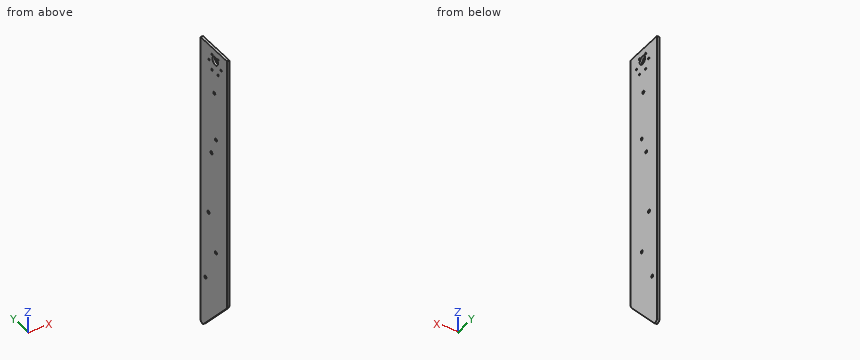
from build123d import *

# Parameters (mm, degrees)
SKETCH_1_R      = 2.5
SKETCH_1_R_2    = 7
SKETCH_1_R_3    = 1.6
EXTRUDE_1_DEPTH = 4


with BuildPart() as part:
    # 草图1 → 凸台-拉伸1 (new body)
    with BuildSketch(Plane.ZY):
        with BuildLine():
            Line((-207.252247772, -7.404631077), (226.406668198, -7.404631077))
            Line((226.406668198, -7.404631077), (226.406668198, 59.595368923))
            Line((226.406668198, 59.595368923), (-273.593331802, 59.595368923))
            ThreePointArc((-273.593331802, 59.595368923), (-277.860990507, 56.662288358), (-276.652116001, 51.626963655))
            Line((-276.652116001, 51.626963655), (-213.943553835, -4.836079331))
            ThreePointArc((-213.943553835, -4.836079331), (-210.835927267, -6.740435342), (-207.252247772, -7.404631077))
        make_face()
        with Locations((-191.007742204, 47.443421044)):
            Circle(SKETCH_1_R, mode=Mode.SUBTRACT)
        with Locations((68.992257796, 20.828748174)):
            Circle(SKETCH_1_R, mode=Mode.SUBTRACT)
        with Locations((38.992257796, 32.145259985)):
            Circle(SKETCH_1_R, mode=Mode.SUBTRACT)
        with Locations((-131.007742204, 20.828748174)):
            Circle(SKETCH_1_R, mode=Mode.SUBTRACT)
        with Locations((207.406668198, 22.602258186)):
            Circle(SKETCH_1_R_2, mode=Mode.SUBTRACT)
        with Locations((148.992257796, 24.828748174)):
            Circle(SKETCH_1_R, mode=Mode.SUBTRACT)
        with Locations((-71.007742204, 39.461771796)):
            Circle(SKETCH_1_R, mode=Mode.SUBTRACT)
        with Locations((213.830061956, 30.756889262)):
            Circle(SKETCH_1_R_3, mode=Mode.SUBTRACT)
        with Locations((200.406668198, 38.506889262)):
            Circle(SKETCH_1_R_3, mode=Mode.SUBTRACT)
        with Locations((186.983274439, 30.756889262)):
            Circle(SKETCH_1_R_3, mode=Mode.SUBTRACT)
        with Locations((186.983274439, 15.256889262)):
            Circle(SKETCH_1_R_3, mode=Mode.SUBTRACT)
        with Locations((200.406668198, 7.506889262)):
            Circle(SKETCH_1_R_3, mode=Mode.SUBTRACT)
        with Locations((213.830061956, 15.256889262)):
            Circle(SKETCH_1_R_3, mode=Mode.SUBTRACT)
    extrude(amount=EXTRUDE_1_DEPTH)


solid = part.part
Could you check a few things on this model? Use its own coordinates, in mm. Round coordinates to 2 decimals unless told otherwise and drop trailing zeros. Write item = value, one per line.
1) I need wall thicknesses on line 1 along Z through (x, y) = (-0.3, 39); line 2 along Z through (x, y) = (-0.2, 20) (3 decimals); line 3 along Z through (x, y) = (-3.3, 17). Which ranges of each line are inside material? Lowest first, please. Write a range as from..to.
Computed:
line_1 = -262.63..-73.46, -68.55..198.88, 201.93..226.41
line_2 = -241.527..-133.366, -128.649..66.634, 71.351..200.908, 213.905..226.407
line_3 = -238.19..203.21, 211.6..226.41
2) I'm going to push flat-ended pins straight in: P1, Ø2, axis at x = -3.5, y = 37.5, coming from the -Z side; P2, Ø4, axis at y = 24.83, z = 148.99, coming from the +X side. Where does each tip first touch, or does it pass through?
Computed:
P1 = -262.07
P2 = through
3) Imagine slicing it at A-A (x = -3.2). Give the number of separate pieces and of enclosed holes in the cut face, and give its area (3 significant figures).
Computed:
separate_pieces = 1
enclosed_holes = 13
area = 31,500 mm2
